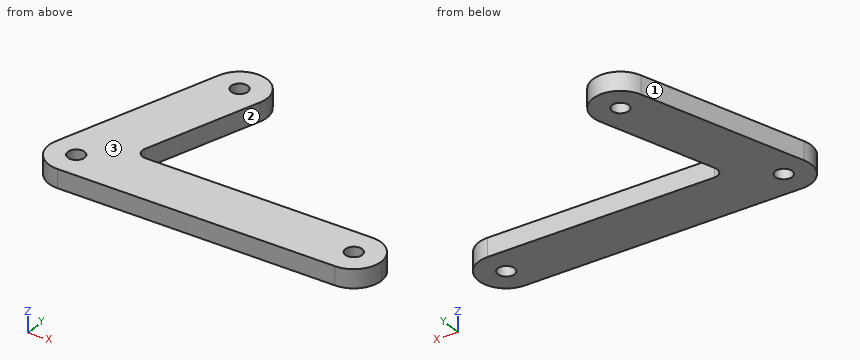
from build123d import *

# Parameters (mm, degrees)
BOSS_EXTRUDE1_DEPTH = 5.08


with BuildPart() as part:
    # Sketch1 → Boss-Extrude1 (new body)
    with BuildSketch(Plane.XY):
        with BuildLine():
            ThreePointArc((50.8526553, 100.196470122), (51.917951715, 93.470453272), (57.985579172, 90.378842665))
            Line((57.985579172, 90.378842665), (133.585579172, 90.378842665))
            ThreePointArc((133.585579172, 90.378842665), (138.888880031, 92.575541806), (141.085579172, 97.878842665))
            ThreePointArc((141.085579172, 97.878842665), (138.888880031, 103.182143524), (133.585579172, 105.378842665))
            Line((133.585579172, 105.378842665), (71.804453654, 105.378842665))
            ThreePointArc((71.804453654, 105.378842665), (69.749550488, 106.425868124), (69.388770103, 108.70374583))
            Line((69.388770103, 108.70374583), (79.55681827, 139.99778028))
            ThreePointArc((79.55681827, 139.99778028), (74.741521855, 149.44833161), (65.290970525, 144.633035196))
            Line((65.290970525, 144.633035196), (50.8526553, 100.196470122))
        make_face()
        with BuildLine():
            ThreePointArc((60.285579172, 97.878842665), (57.985579172, 95.578842665), (55.685579172, 97.878842665))
            ThreePointArc((55.685579172, 97.878842665), (57.985579172, 100.178842665), (60.285579172, 97.878842665))
        make_face(mode=Mode.SUBTRACT)
        with BuildLine():
            ThreePointArc((135.885579172, 97.878842665), (133.585579172, 95.578842665), (131.285579172, 97.878842665))
            ThreePointArc((131.285579172, 97.878842665), (133.585579172, 100.178842665), (135.885579172, 97.878842665))
        make_face(mode=Mode.SUBTRACT)
        with BuildLine():
            ThreePointArc((74.611324385, 141.604668651), (71.713155311, 140.12797775), (70.23646441, 143.026146825))
            ThreePointArc((70.23646441, 143.026146825), (73.134633485, 144.502837725), (74.611324385, 141.604668651))
        make_face(mode=Mode.SUBTRACT)
    extrude(amount=BOSS_EXTRUDE1_DEPTH)


solid = part.part
Could you check a few things on this model? Use its own coordinates, in mm. Face numbers are marked on the shaded views. Round coordinates to 2 decimals unless told otherwise and drop trailing zeros. Order: outer loops, then holes, each group sorted by start corner. A loop starts at its lowest first (then second) coordinate and runs counter-clockwise, first axis right, second up.
(1) If we mould it in two halves opening along Y, with no side actions, what happens to the marked faces 1, 2 and 3? For each: released by +Y, released by -Y, zero draft, split by the parting line, or undercut.
Response values:
face 1: released by +Y
face 2: undercut
face 3: zero draft
(2) I'm going to push flat-ended pins straight in: pin 1 (4 mm diameter, centred on x = 133.59, y = 97.88, fed in from +Z); pin 2 (1.5 mm diameter, centred on x = 88.5, z = 3, fed in from +Y). Where does each tip first touch, or does it pass through?
Response values:
pin 1: passes through
pin 2: stops at y = 105.38
(3) Please list where these lines run through material, in increasing order: line 1 along X through (y, z) = (142.5, 1.05); line 2 along Y through (x, z) = (112.5, 3.95); line 3 along X through (y, z) = (97, 1.3).
Response values:
line 1: x = 64.6 to 70.13, 74.72 to 79.92
line 2: y = 90.38 to 105.38
line 3: x = 50.54 to 55.86, 60.11 to 131.46, 135.71 to 141.03
(4) Imagine slicing it at A-A (z = 3.9). Write out the boundary of the cut face in (x, y), plus the area to 3 significant figures.
Response values:
outline: (50.85, 100.2) arc R7.5 ccw to (57.99, 90.38) - (133.59, 90.38) arc R7.5 ccw to (133.59, 105.38) - (71.8, 105.38) arc R2.54 cw to (69.39, 108.7) - (79.56, 140) arc R7.5 ccw to (65.29, 144.63) - close; hole circle Ø4.6 at (57.99, 97.88); hole circle Ø4.6 at (72.42, 142.32); hole circle Ø4.6 at (133.59, 97.88)
area: 1,940 mm2
(5) Imagine slicing it at C-C (y = 138.5). Write out the boundary of the cut face in (x, z), plus the area to 3 significant figures.
Response values:
outline: (63.3, 0) - (79.07, 0) - (79.07, 5.08) - (63.3, 5.08) - close
area: 80.1 mm2
(6) Imagine slicing it at B-B (x = 121.5). Write out the boundary of the cut face in (y, z), plus the area to 3 significant figures.
Response values:
outline: (90.38, 0) - (105.38, 0) - (105.38, 5.08) - (90.38, 5.08) - close
area: 76.2 mm2
